Part model, mm, in its own coordinate system. A direction names the side the tool comes from. Coordinates: 2 decimals unless noted, no trailing zeros. Loops run counter-clockwise (first coordinate to the right, second up) from the corner with the lowest first, then second, coordinate; pieces in that order, holes last. Notation, with made-up numbers: M 27.5,31.25 L 55.5,31.25 A7 cw 55.5,36.25 Z; hole C 57,80.5 d5. An arc over 180 degrees is marked long. Answer as a JSON object with one key per item and string values. Group by question number.
1. Saw through at A-A on z = 5. Write the cut outline in (x, y).
2. Mould opens along Y. For faces 3 (the face through (-5.994, 0.264, 2.493)), 4 (the face through (-3, 0, 4)), 5 (the face through (1, -4, 3)) say: released by +Y, released by -Y, zero draft, split by the parting line, or undercut.
3. 3-axis set-ups, long thin cutter, end or side, ignore diameter. For faces 1 (the face through (5, -5, 2)), 2 (the face through (0, 0, 0)): which of +Z, -Z, +X, -X, +Y, -Y reach the whole face in a straight line?
4. Drop flat-ended pins along their axis: pin 1 Ø2 at (x, y) = (5, -5.5) entering from +Z; pin 2 Ø3 at (x, z) = (9, 1) entering from -Y. Give the stop position or say it passes through.
5. Saw through at B-B on x = 0. Write the cut outline in (y, z).
6. Saw through at D-D on z = 1.45. Write the cut outline in (x, y).
7. Drill centre lines: L1, parallel to Y at x = 0, z = 5.15; L2, parallel to X at y = 4.25, z = 0.45; L3, parallel to Z at x = -9.75, y = 1.75. Where is each one in solid material? Low to high.
from build123d import *

# Parameters (mm, degrees)
F0_R     = 11.5
F1_DEPTH = 2
F2_R     = 1
F3_R     = 3.85
F3_R_2   = 3
F4_DEPTH = 4
F3_R_3   = 6
F5_DEPTH = 1


with BuildPart() as f1:
    # F0 (on Top) → F1 (new body)
    with BuildSketch(Plane.XY):
        Circle(F0_R)
    extrude(amount=F1_DEPTH)

    # F2
    f2_edges = [f1.edges().sort_by_distance(p)[0] for p in [
        (-11.5, 0, 0),
    ]]
    fillet(f2_edges, radius=F2_R)

    # F3 (on face) → F4 (join)
    with BuildSketch(Plane.XY.offset(2)):
        Circle(F3_R)
        Circle(F3_R_2, mode=Mode.SUBTRACT)
    extrude(amount=F4_DEPTH)

    # F3 (on face) → F5 (join)
    with BuildSketch(Plane.XY.offset(2)):
        Circle(F3_R_3)
        Circle(F3_R, mode=Mode.SUBTRACT)
    extrude(amount=F5_DEPTH)


solid = f1.part
Outcome:
{
 "1": {"outline": "C 0,0 d7.7; hole C 0,0 d6"},
 "2": {"face 3": "split by the parting line", "face 4": "undercut", "face 5": "zero draft"},
 "3": {"face 1": "+Z", "face 2": "-Z, +X, -X, +Y, -Y"},
 "4": {"pin 1": "stops at z = 2", "pin 2": "stops at y = -8.72"},
 "5": {"outline": "M -11.5,1 A1 ccw -10.5,0 L 10.5,0 A1 ccw 11.5,1 L 11.5,2 L 6,2 L 6,3 L 3.85,3 L 3.85,6 L 3,6 L 3,2 L -3,2 L -3,6 L -3.85,6 L -3.85,3 L -6,3 L -6,2 L -11.5,2 Z"},
 "6": {"outline": "C 0,0 d23"},
 "7": {"L1": "y = -3.85 to -3, 3 to 3.85", "L2": "x = -10.51 to 10.51", "L3": "z = 0 to 2"}
}
